Design review of the part built by this model. Coordinates are the model's own, in mm. A direction names the side the tool comes from. Coordinates: 2 decimals unless noted, no trailing zeros. Write each loop counter-clockwise with the first axis right and the second up, starting at its lowest first coordinate (ties: lowest second). Pieces come first, ordered by that corner, then holes. Notation, with made-up numbers: M 66.25,52.25 L 123.25,52.25 A10 ccw 123.25,56.25 Z; hole C 50.25,-19 d2. An arc over 180 degrees is marked long. Write item = value, one per line.
```python
from build123d import *

# Parameters (mm, degrees)
F1_DEPTH = 3


with BuildPart() as f1:
    # F0 (on Right) → F1 (new body)
    with BuildSketch(Plane.YZ):
        with BuildLine():
            Line((-5.053473, -29.057488), (55.02674, -29.057488))
            Line((55.02674, -29.057488), (55.02674, -20.354279))
            ThreePointArc((55.02674, -20.354279), (48.692747, -9.279821), (35.93583, -9.124332))
            Line((35.93583, -9.124332), (35.93583, -24.28476))
            Line((35.93583, -24.28476), (32.566845, -24.28476))
            Line((32.566845, -24.28476), (32.566845, -10.762674))
            Line((32.566845, -10.762674), (-5.053473, -29.057488))
        make_face()
    extrude(amount=F1_DEPTH)


solid = f1.part
```
Q1. Machinability: for faces 5 (the flat face through (1, 35.936, -17)), 6 (the flat face through (0, 31, -21)), which of the approach directions +Z, -Z, +X, -X, +Y, -Y give a long, thin tool a straight path to every point of the face, cutting with its end or side? Answer none if there is none.
Check result:
face_5 = +Z, +X, -X
face_6 = +Z, -Z, -X, +Y, -Y
Q2. Consider section A-A, the plane z = -15.25. State the section outline as (x, y) points, and give its area (3 significant figures).
Check result:
outline = M 0,23.34 L 3,23.34 L 3,32.57 L 0,32.57 Z; M 0,35.94 L 3,35.94 L 3,53.97 L 0,53.97 Z
area = 81.8 mm²
Q3. The part is to be moulded in two halves that separate along Y. For faces 1 (the cylindrical face through (1.479, 48.853, -9.376)), 2 (the flat face through (1, 32.567, -18)), 3 (the flat face through (1, 34, -24.285)), 4 (the flat face through (1, 25, -29.057)), say which applies: +Y half, -Y half, draft (parallel to the pull), parting line (faces both ways), or undercut.
Check result:
face_1 = parting line
face_2 = undercut
face_3 = undercut
face_4 = draft
Q4. Consider section D-D, the plane y = 18. State the section outline as (x, z) points.
Check result:
outline = M 0,-29.06 L 3,-29.06 L 3,-17.85 L 0,-17.85 Z
Q5. Consider section C-C, the plane z = -21.25. State the section outline as (x, y) points.
Check result:
outline = M 0,11 L 3,11 L 3,32.57 L 0,32.57 Z; M 0,35.94 L 3,35.94 L 3,55.03 L 0,55.03 Z
Q6. Consider section B-B, the plane x = 0.5. State the section outline as (y, z) points, and give its area (3 significant figures).
Check result:
outline = M -5.05,-29.06 L 55.03,-29.06 L 55.03,-20.35 A12.85 ccw 35.94,-9.12 L 35.94,-24.28 L 32.57,-24.28 L 32.57,-10.76 Z
area = 733 mm²
Q7. For P1, Ø1.5, axis at x = 1, z = -16.5, coming from the -Y side; P2, Ø0.9, axis at x = 1.5, z = -19, coming from the +Y side; P3, Ø1.5, axis at x = 2, y = 34, coming from the +Z side, all flat-tipped, find the tip position at first contact; note any pin that passes through.
Check result:
P1 = 19.23
P2 = 54.99
P3 = -24.28
Q8. Wall thickness on line 1 (Y direction, x = 0.8, z = -11.5); line 2 (Y direction, x = 2.15, z = -14.25); line 3 (Z direction, x = 0.4, y = 42.5): over which ranges is each line inside the solid? List them lowest first.
Check result:
line_1 = 31.05 to 32.57, 35.94 to 51.49
line_2 = 25.4 to 32.57, 35.94 to 53.48
line_3 = -29.06 to -7.51
